Part print with two shaded views. Sizes in mm from the minimum x, y, z corner. A direction names the side the tool comes from. Coordinates: 2 decimals unless noted, no trailing zeros. Loops run counter-clockwise (first coordinate to the right, second up) from the corner with the lowest first, then second, coordinate; pieces in that order, holes last. Notation, with made-up numbers: (-13, -13.75) -> (-5, -13.75) arc R24 cw to (-5, 12.25) -> close; hole circle Ø5 at (48, -24). An arc over 180 degrees is marked (long way). Return JSON: item names as keys, results as strings. Group by question number.
(1) Probe L1, parallel to Y at x = 26.5, z = 8 (1 decimal); L2, parallel to X at y = 20, z = 11.75 (1 decimal); L3, parallel to Y at x = 98, z = 4.5 (1 decimal). List the from-to ranges inside material, lowest first.
(2) Saw through at C-C on z = 6.5. Write the cut outline in (x, y) (1 decimal), then the cut area to 3 significant figures.
(3) Tool access for the marked faces 4 and 5: list every direction of +Z, -Z, +X, -X, +Y, -Y with a clear straight run to the whole face (end or side of a thin tool).
(4) Saw through at D-D on x = 38. Write the cut outline in (y, z) (1 decimal).
(5) Saw through at B-B on y = 78.5. Write the cut outline in (x, z) (1 decimal).
(6) Mould opens along Y. For the marked faces 1, 2 and 3 say: pulls with the +Y half, pulls with the -Y half, needs draft (parallel to the pull), parting line crosses it, or undercut.
(7) Saw through at A-A on x = 102. Write the cut outline in (y, z) (1 decimal).
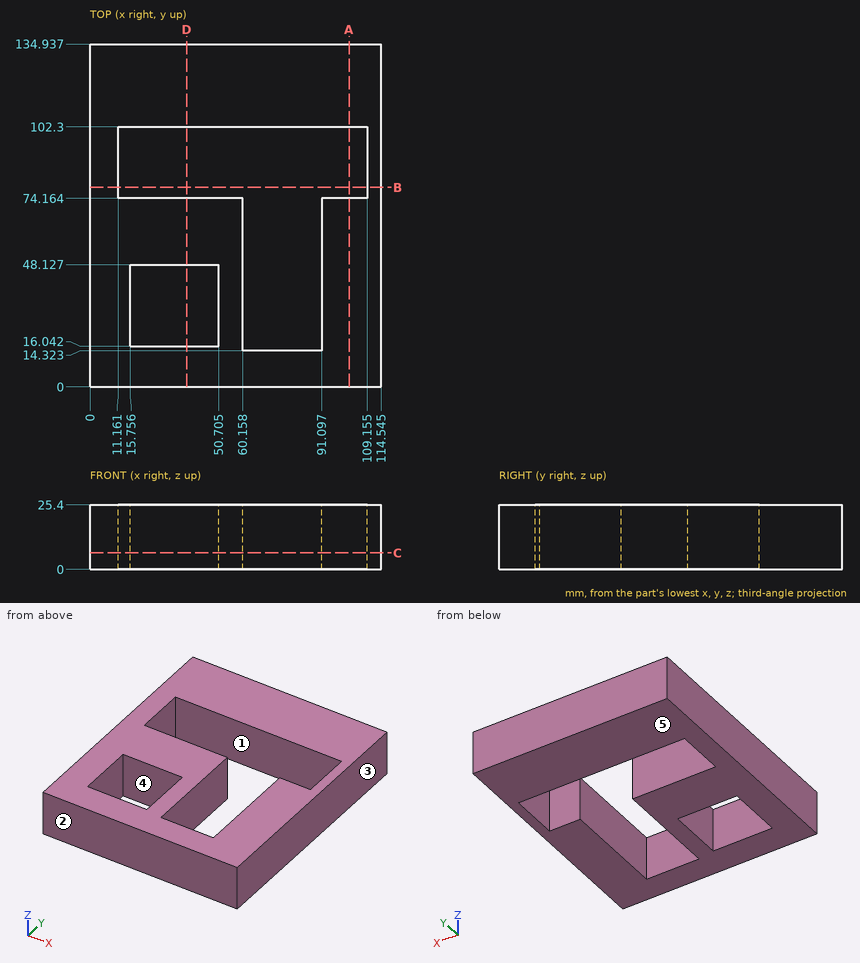
Geometry results:
{
 "1": {"L1": "0 to 16, 48.1 to 74.2, 102.3 to 134.9", "L2": "0 to 15.8, 50.7 to 60.2, 91.1 to 114.5", "L3": "0 to 74.2, 102.3 to 134.9"},
 "2": {"outline": "(0, 0) -> (114.5, 0) -> (114.5, 134.9) -> (0, 134.9) -> close; hole (11.2, 74.2) -> (60.2, 74.2) -> (60.2, 14.3) -> (91.1, 14.3) -> (91.1, 74.2) -> (109.2, 74.2) -> (109.2, 102.3) -> (11.2, 102.3) -> close; hole (15.8, 16) -> (50.7, 16) -> (50.7, 48.1) -> (15.8, 48.1) -> close", "area": "9,730 mm²"},
 "3": {"face 4": "+Z, -Z", "face 5": "-Z, +X, -X, +Y, -Y"},
 "4": {"outline": "(0, 0) -> (16, 0) -> (16, 25.4) -> (0, 25.4) -> close; (48.1, 0) -> (74.2, 0) -> (74.2, 25.4) -> (48.1, 25.4) -> close; (102.3, 0) -> (134.9, 0) -> (134.9, 25.4) -> (102.3, 25.4) -> close"},
 "5": {"outline": "(0, 0) -> (11.2, 0) -> (11.2, 25.4) -> (0, 25.4) -> close; (109.2, 0) -> (114.5, 0) -> (114.5, 25.4) -> (109.2, 25.4) -> close"},
 "6": {"face 1": "undercut", "face 2": "pulls with the -Y half", "face 3": "needs draft"},
 "7": {"outline": "(0, 0) -> (74.2, 0) -> (74.2, 25.4) -> (0, 25.4) -> close; (102.3, 0) -> (134.9, 0) -> (134.9, 25.4) -> (102.3, 25.4) -> close"}
}
